```python
from build123d import *

# Parameters (mm, degrees)
SKETCH_1_W      = 60
SKETCH_1_H      = 12
SKETCH_1_R      = 1.5
EXTRUDE_1_DEPTH = 3.85
FILLET_1_R      = 6


with BuildPart() as part:
    # 草图1 → 凸台-拉伸1 (new body)
    with BuildSketch(Plane.XY):
        with Locations((5, 0)):
            Rectangle(SKETCH_1_W, SKETCH_1_H)
        with Locations(Location((-20, 0, 0), (0, 0, 180))):
            Circle(SKETCH_1_R, mode=Mode.SUBTRACT)
        with Locations(Location((30, 0, 0), (0, 0, 180))):
            Circle(SKETCH_1_R, mode=Mode.SUBTRACT)
    extrude(amount=EXTRUDE_1_DEPTH)

    # 圆角1
    fillet_1_edges = [part.edges().sort_by_distance(p)[0] for p in [
        (-25, -6, 1.925),
        (-25, 6, 1.925),
    ]]
    fillet(fillet_1_edges, radius=FILLET_1_R - 0.0001)  # a hair under: the kernel refuses the full size


solid = part.part
```
Input: part model. Units: mm. Frame: model coordinates. Give positions to 0.01 mm unless a question says otherwise; leave off trailing zeros. Loops run counter-clockwise (first coordinate to the right, second up) from the corner with the lowest first, then second, coordinate; pieces in that order, holes last.
1) Section query B-B on x = -20. Return the cut outline in (y, z).
A:
outline: (-5.92, 0) - (-1.5, 0) - (-1.5, 3.85) - (-5.92, 3.85) - close; (1.5, 0) - (5.92, 0) - (5.92, 3.85) - (1.5, 3.85) - close
2) Line query: L1, parallel to X at y = 0.5, z = 1.7; L2, parallel to Y at x = -20, z = 1.65; L3, parallel to X at y = 3.25, z = 3.65. Output: solid intervals per line, ascending.
A:
L1: x = -24.98 to -21.41, -18.59 to 28.59, 31.41 to 35
L2: y = -5.92 to -1.5, 1.5 to 5.92
L3: x = -24.04 to 35
3) Mould query, pull axis Y, two halves, no side actions, for faces 1 (the cylindrical face through (31.5, -0.07, 1.9)), 2 (the flat face through (5, 0, 0)), 3 (the flat face through (8, 6, 2)), 4 (the cylindrical face through (-18.5, -0.07, 1.9)). Classes: released by +Y, released by -Y, zero draft, split by the parting line, or undercut.
A:
face 1: undercut
face 2: zero draft
face 3: released by +Y
face 4: undercut
4) Section query A-A on z = 0.9. Count the separate pieces of the cut face and the enclosed holes in it, and give its area (3 significant figures).
A:
separate pieces: 1
enclosed holes: 2
area: 690 mm2
5) Section query D-D on y = 4.75. Return the cut outline in (x, z).
A:
outline: (-22.67, 0) - (35, 0) - (35, 3.85) - (-22.67, 3.85) - close
6) Section query C-C on y = -4. Return the cut outline in (x, z), and give its area (3 significant figures).
A:
outline: (-23.47, 0) - (35, 0) - (35, 3.85) - (-23.47, 3.85) - close
area: 225 mm2
7) Contact query for a flat-ended pin moving along its axis: pin 1 (1 mm diameter, centred on x = 18.5, y = 2, fed in from -Z). Output: stop coordinate, or through.
A:
pin 1: stops at z = 0
